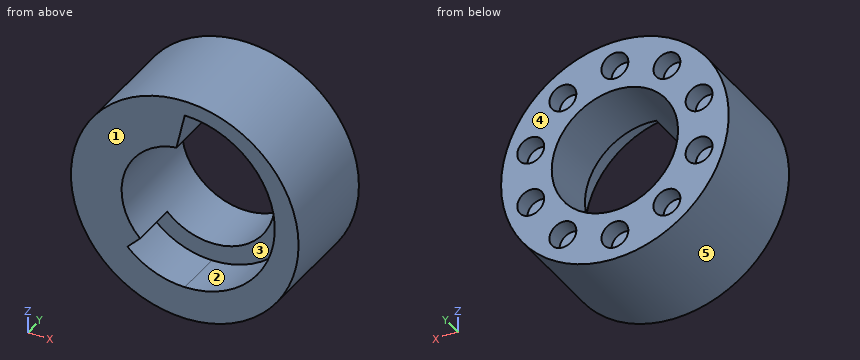
```python
from build123d import *

# Parameters (mm, degrees)
F0_R            = 12.7
F0_R_2          = 7.05
F1_DEPTH        = 12
F3_DEPTH        = 5.4
F4_R            = 1.5
F5_DEPTH        = 2
F5_COPIES_COUNT = 10


# Not quite as in the source:
# - a pattern or mirror of a feature is missing from the dataset's text; its kind, count and spacing are read off the source's solid


with BuildPart() as f1:
    # F0 (on Front) → F1 (new body)
    with BuildSketch(Plane.XZ):
        Circle(F0_R)
        Circle(F0_R_2, mode=Mode.SUBTRACT)
    extrude(amount=F1_DEPTH)

    # F2 (on face) → F3 (cut)
    with BuildSketch(Plane.XZ.offset(12)):
        with BuildLine():
            Line((-4.9851028074, -4.9851028074), (-6.3993163697, -6.3993163697))
            ThreePointArc((-6.3993163697, -6.3993163697), (-3.4632850629, -8.3611097692), (0, -9.05))
            ThreePointArc((0, -9.05), (10.05, 1), (0, 11.05))
            Line((0, 11.05), (-0.9218489985, 6.9894702535))
            ThreePointArc((-0.9218489985, 6.9894702535), (6.6761231195, -2.2653653334), (-4.9851028074, -4.9851028074))
        make_face()
    extrude(amount=-F3_DEPTH, mode=Mode.SUBTRACT)

    # F4 (on face) → F5 (cut)
    with BuildSketch(Plane(origin=(0, 0, 0), x_dir=(-1, 0, 0), z_dir=(0, 1, 0))):
        with Locations((0, 9.875)):
            Circle(F4_R)
    f5 = extrude(amount=-F5_DEPTH, mode=Mode.SUBTRACT)

    # F5_copies: F5 ×10 about axis
    f5_copies_axis = Axis((0, 0, 0), (0, 1, 0))
    for i in range(1, F5_COPIES_COUNT):
        add(f5.rotate(f5_copies_axis, i * 360 / F5_COPIES_COUNT), mode=Mode.SUBTRACT)


solid = f1.part
```
Design review of the part built by this model. Coordinates are the model's own, in mm. Face numbers are marked on the shaded views. A direction names the side the tool comes from. Give positions to 0.01 mm unless a question says otherwise; leave off trailing zeros. Write each loop counter-clockwise with the first axis right and the second up, starting at its lowest first coordinate (ties: lowest second). Pieces come first, ordered by that corner, then holes. Notation, with made-up numbers: (-13, -28) -> (-7, -28) arc R26 ccw to (-7, -11) -> close; hole circle Ø6 at (-10, 11). An arc over 180 degrees is marked (long way). Answer in a Markdown table with one row per item.
(1) To check wall thickness, follow probe 1 along Z at (x, y) = (0, -1.1) (3 decimals); probe 2 along Z at (x, y) = (-5.5, -9.75); probe 3 along X at (y, z) = (-5.5, 6). State the ranges of each line that lie inside material, in increasing order.
Results:
| item | result |
|---|---|
| probe 1 | -12.7 to -11.375, -8.375 to -7.05, 7.05 to 8.375, 11.375 to 12.7 |
| probe 2 | -11.45 to -7.19, -5.5 to -4.41, 4.41 to 11.45 |
| probe 3 | -11.19 to -3.7, 3.7 to 11.19 |
(2) Consider section C-C (y = -6). State the section outline as (x, z) points.
Results:
| item | result |
|---|---|
| outline | circle Ø25.4 at (0, 0); hole circle Ø14.1 at (0, 0) |
(3) Consider section A-A (z = 0). State the section outline as (x, y) points, then the cut area to 3 significant figures.
Results:
| item | result |
|---|---|
| outline | (-12.7, -12) -> (-7.05, -12) -> (-7.05, 0) -> (-12.7, 0) -> close; (7.05, -6.6) -> (10, -6.6) -> (10, -12) -> (12.7, -12) -> (12.7, 0) -> (7.05, 0) -> close |
| area | 120 mm2 |
(4) Consider section B-B (x = 3.25). State the section outline as (y, z) points, then the cut area to 3 significant figures.
Results:
| item | result |
|---|---|
| outline | (-12, -12.28) -> (0, -12.28) -> (0, -6.26) -> (-6.6, -6.26) -> (-6.6, -8.51) -> (-12, -8.51) -> close; (-12, 10.51) -> (-6.6, 10.51) -> (-6.6, 6.26) -> (0, 6.26) -> (0, 12.28) -> (-12, 12.28) -> close |
| area | 109 mm2 |
(5) For the marked faces 1 and 2, list the 3-axis set-ups (+Z, -Z, +X, -X, +Y, -Y) from which the entire face can be reached by the end or side of a thin tool; tool diameter is ignored.
Results:
| item | result |
|---|---|
| face 1 | +Z, -Z, +X, -X, -Y |
| face 2 | -Y |
(6) Clearance check with flat-ended pins moving along their axes: pin 1 (0.9 mm diameter, centred on x = 9.5, z = 2.5, fed in from +Y); pin 2 (4 mm diameter, centred on y = -5, z = 6.5, fed in from +X); pin 3 (3.5 mm diameter, centred on x = 9.39, z = 3.05, fed in from +Y); pin 4 (2 mm diameter, centred on y = -3, z = 6.5, fed in from -X). State where each tip first meets the part, or that it passes through.
Results:
| item | result |
|---|---|
| pin 1 | y = -2 |
| pin 2 | x = 11.88 |
| pin 3 | y = 0 |
| pin 4 | x = -11.45 |
(7) Mouldability with a two-part tool opening along Z and no side actions: class the marked faces 3, 4 and 5 as +Z half, -Z half, draft (parallel to the pull), parting line (faces both ways), or undercut.
Results:
| item | result |
|---|---|
| face 3 | undercut |
| face 4 | draft |
| face 5 | parting line |
(8) Consider section D-D (x = 9.5). State the section outline as (y, z) points, then the cut area to 3 significant figures.
Results:
| item | result |
|---|---|
| outline | (-12, -8.43) -> (0, -8.43) -> (0, -4.55) -> (-2, -4.55) -> (-2, -1.56) -> (0, -1.56) -> (0, 1.56) -> (-2, 1.56) -> (-2, 4.55) -> (0, 4.55) -> (0, 8.43) -> (-12, 8.43) -> (-12, 4.28) -> (-6.6, 4.28) -> (-6.6, -2.28) -> (-12, -2.28) -> close |
| area | 155 mm2 |
